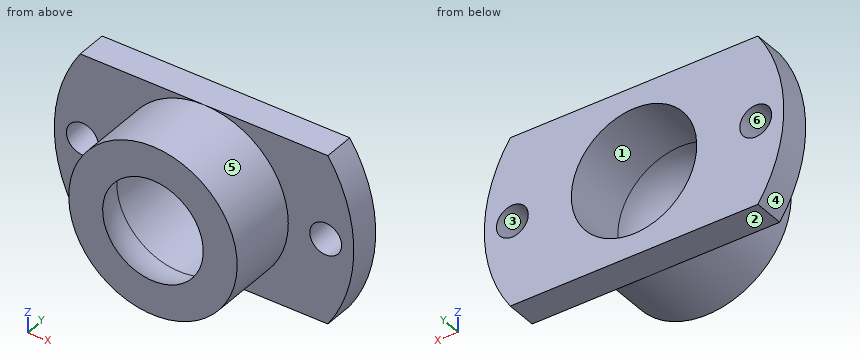
```python
from build123d import *

# Parameters (mm, degrees)
CIRPATTERN2_COUNT  = 2
SKETCH5_W          = 50.426982916
SKETCH5_H          = 37.261009064
SKETCH5_W_2        = 37.991098709
SKETCH5_H_2        = 18
CUT_EXTRUDE1_DEPTH = 4.3


with BuildPart() as part:
    # Sketch1 → Revolve1 (revolve)
    with BuildSketch(Plane(origin=(0, 0, 0), x_dir=(0, 0, -1), z_dir=(1, 0, 0))):
        with BuildLine():
            ThreePointArc((-6.7, 0), (-6.360114404, -2.10688034), (-5.37494186, -4))
            Line((-5.37494186, -4), (-9, -4))
            Line((-9, -4), (-9, 3.7))
            Line((-9, 3.7), (-16, 3.7))
            Line((-16, 3.7), (-16, 7))
            Line((-16, 7), (-6.7, 7))
            Line((-6.7, 7), (-6.7, 0))
        make_face()
    revolve(axis=Axis((0, 0, 0), (0, 1, 0)))

    # Sketch3 → M3 Clearance Hole1 (revolve, cut)
    with BuildSketch(Plane(origin=(-13, 3.7, 0), x_dir=(0, 0, -1), z_dir=(1, 0, 0))):
        Polygon((0, 0), (0, 11.021463052), (1.7, 10), (1.7, 0), align=None)
    m3_clearance_hole1 = revolve(axis=Axis((-13, -2.65, 0), (0, 1, 0)), mode=Mode.SUBTRACT)

    # CirPattern2: M3 Clearance Hole1 ×2 about axis
    cirpattern2_axis = Axis((0, 0, 0), (0, 1, 0))
    for i in range(1, CIRPATTERN2_COUNT):
        add(m3_clearance_hole1.rotate(cirpattern2_axis, i * 360 / CIRPATTERN2_COUNT), mode=Mode.SUBTRACT)

    # Sketch5 → Cut-Extrude1 (cut, through all)
    with BuildSketch(Plane.XZ.offset(-3.7)):
        with Locations((1.488148737, -0.857756759)):
            Rectangle(SKETCH5_W, SKETCH5_H)
        with Locations((1.919239442, 0)):
            Rectangle(SKETCH5_W_2, SKETCH5_H_2, mode=Mode.SUBTRACT)
    extrude(amount=-CUT_EXTRUDE1_DEPTH, mode=Mode.SUBTRACT)


solid = part.part
```
Geometry: final body of the model. Coordinates: model frame, mm. Face numbers are marked on the shaded views. A direction names the side the tool comes from. Round coordinates to 2 decimals unless told otherwise and drop trailing zeros. Order: outer loops, then holes, each group sorted by start corner. A loop starts at its lowest first (then second) coordinate and runs counter-clockwise, first axis right, second up. Notation, with made-up numbers: M 5,-24.75 L 61,-24.75 A9 cw 61,-18.75 Z; hole C 87.5,-27 d10. An arc over 180 degrees is marked long. Use one line per item in the form item = value. Start each with the question number.
Q1. Mould query, pull axis X, two halves, no side actions, for the marked faces 3, 4, 5 and 6. Classes: +X half, -X half, draft (parallel to the pull), parting line (faces both ways), or undercut.
Q2. Cut plane A-A (z = 0.75). Return loops of the section in (x, y), and give its area (3 significant figures).
Q3. Pin query (flat end, axial travel): pin 1 Ø4.5 at (x, z) = (-13, 0) entering from -Y. Return the tip coordinate at first contact, or that it passes through.
Q4. Cut plane B-B (x = 2). Return loops of the section in (y, z), and give its area (3 significant figures).
Q5. Cut plane C-C (y = 4.75). Return loops of the section in (x, z).
Q6. Cut plane D-D (z = -4.5). Return loops of the section in (x, y).
Q7. Access query for the marked faces 1 and 2. Directions: +Z, -Z, +X, -X, +Y, -Y. A direction counts if a zero-diameter tool reaches every point of the face in a straight line with its end or side. Return the directions, or none.
Q8. Material intervals for line 1 (X direction, y = 5.3, z = 0); line 2 (Z direction, x = -13, y = 5.05); line 3 (X direction, y = 6.25, z = -1.5), sorted ascending. Write a range as [from, to].
Geometry results:
q1.face_3 = undercut
q1.face_4 = -X half
q1.face_5 = parting line
q1.face_6 = undercut
q2.outline = M -15.98,3.7 L -14.53,3.7 L -14.53,7 L -15.98,7 Z; M -11.47,3.7 L -8.97,3.7 L -8.97,-4 L -5.32,-4 A6.66 cw -6.66,0 L -6.66,7 L -11.47,7 Z; M 5.32,-4 L 8.97,-4 L 8.97,3.7 L 11.47,3.7 L 11.47,7 L 6.66,7 L 6.66,0 A6.66 cw Z; M 14.53,3.7 L 15.98,3.7 L 15.98,7 L 14.53,7 Z
q2.area = 80.4 mm^2
q3.pin_1 = 3.7
q4.outline = M -4,-8.77 L 3.7,-8.77 L 3.7,-9 L 7,-9 L 7,-6.39 L 0,-6.39 A6.39 cw -4,-4.99 Z; M -4,4.99 A6.39 cw 0,6.39 L 7,6.39 L 7,9 L 3.7,9 L 3.7,8.77 L -4,8.77 Z
q4.area = 57.4 mm^2
q5.outline = M -13.23,-9 L 13.23,-9 A16 ccw 13.23,9 L -13.23,9 A16 ccw Z; hole C -13,0 d3.4; hole C 0,0 d13.4; hole C 13,0 d3.4
q6.outline = M -15.35,3.7 L -7.79,3.7 L -7.79,-4 L -2.94,-4 A4.96 cw -4.96,0 L -4.96,7 L -15.35,7 Z; M 2.94,-4 L 7.79,-4 L 7.79,3.7 L 15.35,3.7 L 15.35,7 L 4.96,7 L 4.96,0 A4.96 cw Z
q7.face_1 = +Y
q7.face_2 = -Z, +X, -X, +Y, -Y
q8.line_1 = [-16, -14.7], [-11.3, -6.7], [6.7, 11.3], [14.7, 16]
q8.line_2 = [-9, -1.7], [1.7, 9]
q8.line_3 = [-15.93, -13.8], [-12.2, -6.53], [6.53, 12.2], [13.8, 15.93]
